The listing builds one solid part. Answer for the finished solid, in the listing's coordinates (mm). Coordinates: 2 decimals unless noted, no trailing zeros. Write each loop counter-clockwise with the first axis right and the second up, starting at its lowest first coordinate (ties: lowest second). Pieces come first, ordered by that corner, then holes.
from build123d import *

# Parameters (mm, degrees)
SKETCH1_W           = 38.1
SKETCH1_H           = 101.6
SKETCH1_R           = 3.175
SKETCH1_R_2         = 9.525
BOSS_EXTRUDE1_DEPTH = 1.143
CHAMFER1_SIZE       = 10.16
FILLET1_R           = 6.35
SKETCH2_W           = 38.1
SKETCH2_H           = 6.35
CUT_EXTRUDE1_DEPTH  = 55.302562518
FILLET2_R           = 6.35


with BuildPart() as part:
    # Sketch1 → Boss-Extrude1 (new, symmetric)
    with BuildSketch(Plane.XY):
        Rectangle(SKETCH1_W, SKETCH1_H)
        with Locations((0, -31.75)):
            Circle(SKETCH1_R, mode=Mode.SUBTRACT)
        with Locations((0, 6.35)):
            Circle(SKETCH1_R, mode=Mode.SUBTRACT)
        with Locations((0, 38.1)):
            Circle(SKETCH1_R_2, mode=Mode.SUBTRACT)
    extrude(amount=BOSS_EXTRUDE1_DEPTH, both=True)

    # Chamfer1
    chamfer1_edges = [part.edges().sort_by_distance(p)[0] for p in [
        (-19.05, 50.8, 0),
        (19.05, 50.8, 0),
    ]]
    chamfer(chamfer1_edges, length=CHAMFER1_SIZE)

    # Fillet1
    fillet1_edges = [part.edges().sort_by_distance(p)[0] for p in [
        (-19.05, 40.64, 0),
        (8.89, 50.8, 0),
        (-8.89, 50.8, 0),
        (19.05, 40.64, 0),
        (19.05, -50.8, 0),
        (-19.05, -50.8, 0),
    ]]
    fillet(fillet1_edges, radius=FILLET1_R)

    # Sketch2 → Cut-Extrude1 (cut, through all)
    with BuildSketch(Plane.XY.offset(1.143)):
        with Locations((0, -47.625)):
            Rectangle(SKETCH2_W, SKETCH2_H)
    extrude(amount=-CUT_EXTRUDE1_DEPTH, mode=Mode.SUBTRACT)

    # Fillet2
    fillet2_edges = [part.edges().sort_by_distance(p)[0] for p in [
        (-19.05, -44.45, 0),
        (19.05, -44.45, 0),
    ]]
    fillet(fillet2_edges, radius=FILLET2_R)


solid = part.part
1. Section A-A on x = 0 is taken. Give the vertices of the cut face in (y, z) (3 decimals).
Results found:
outline: (-44.45, -1.143) - (-34.925, -1.143) - (-34.925, 1.143) - (-44.45, 1.143) - close; (-28.575, -1.143) - (3.175, -1.143) - (3.175, 1.143) - (-28.575, 1.143) - close; (9.525, -1.143) - (28.575, -1.143) - (28.575, 1.143) - (9.525, 1.143) - close; (47.625, -1.143) - (50.8, -1.143) - (50.8, 1.143) - (47.625, 1.143) - close
2. Section D-D on x = -7.5 is taken. Give the vertices of the cut face in (y, z).
Results found:
outline: (-44.45, -1.14) - (32.23, -1.14) - (32.23, 1.14) - (-44.45, 1.14) - close; (43.97, -1.14) - (50.68, -1.14) - (50.68, 1.14) - (43.97, 1.14) - close
3. A flat-ended cylindrical pin translates along its axis: P1, Ø10, axis at x = 0, y = -31.75, coming from the +Z side. Find the tip coordinate at first contact, or state that the pin passes through.
Results found:
P1: stops at z = 1.14
4. Section B-B on y = 6.35 is taken. Give the vertices of the cut face in (x, z) (3 decimals).
Results found:
outline: (-19.05, -1.143) - (-3.175, -1.143) - (-3.175, 1.143) - (-19.05, 1.143) - close; (3.175, -1.143) - (19.05, -1.143) - (19.05, 1.143) - (3.175, 1.143) - close
5. Section C-C on z = -0.65 is taken. Give the vertices of the cut face in (x, y) (3 decimals).
Results found:
outline: (-19.05, -38.1) arc R6.35 ccw to (-12.7, -44.45) - (12.7, -44.45) arc R6.35 ccw to (19.05, -38.1) - (19.05, 38.01) arc R6.35 ccw to (17.19, 42.5) - (10.75, 48.94) arc R6.35 ccw to (6.26, 50.8) - (-6.26, 50.8) arc R6.35 ccw to (-10.75, 48.94) - (-17.19, 42.5) arc R6.35 ccw to (-19.05, 38.01) - close; hole circle Ø19.05 at (0, 38.1); hole circle Ø6.35 at (0, -31.75); hole circle Ø6.35 at (0, 6.35)
6. Find the intervals of material crossed by L1, parallel to Y at x = 0, z = 0.35 (3 decimals); L2, parallel to Y at x = 7, z = -0.5; L3, parallel to X at y = 46.5, z = -0.8, in increasing order.
Results found:
L1: y = -44.45 to -34.925, -28.575 to 3.175, 9.525 to 28.575, 47.625 to 50.8
L2: y = -44.45 to 31.64, 44.56 to 50.76
L3: x = -13.19 to -4.49, 4.49 to 13.19
7. For a pull along Y with two mould halves and no side action, classify faces 1 (the flat face through (-19.05, -1, 0)), 2 (the cylindrical face through (-8.722, 50.303, -0.016)), 3 (the cylindrical face through (-1.24, 47.544, -0.016)), 4 (the cylindrical face through (1.707, 9.027, -0.016)) as pulls with the +Y half, pulls with the -Y half, needs draft (parallel to the pull), parting line crosses it, or undercut.
Results found:
face 1: needs draft
face 2: pulls with the +Y half
face 3: undercut
face 4: undercut
